Can you work these out from the model? Positions are in its coordinate system, mm. A direction names the side the tool comes from. Coordinates: 2 decimals unless noted, no trailing zeros. Order: outer loops, then holes, each group sorted by start corner. A loop starts at its lowest first (then second) coordinate and runs counter-clockwise, first axis right, second up. Notation, with made-up numbers: (-37.75, -24) - (20.25, -24) arc R21 ccw to (20.25, -7) - close; hole circle Ø4 at (74, 24). An arc over 180 degrees is marked (long way). Return JSON: item names as keys, results as strings. Group by question number.
1) Imagine slicing it at D-D (y = 0.75). Write out the boundary of the cut face in (x, z), and give its area (3 significant figures).
2) Imagine slicing it at C-C (z = 3.25). Write out the boundary of the cut face in (x, y), and give its area (3 significant figures).
3) If I drill on line 1 along X through (y, z) = (-4.25, 4.5); line 2 along Y through (x, z) = (-1.5, 6.75), over which ranges is the centre line in solid material (lowest first)?
4) For pin 1 Ø2.5 at (y, z) = (0, 3) entering from -X; pin 2 Ø0.6 at (x, y) = (6.5, 0) entering from +Z; pin 3 Ø4 at (x, z) = (2, 1.5) entering from -Y; pin 4 Ø2.5 at (y, z) = (-1.5, 3) entering from +X, each with a flat end and sliding along its axis, tell me the tip position at first contact or that it passes through.
5) Which directions (+Z, -Z, +X, -X, +Y, -Y) give clear straight access to the entire face, cutting with the end or side of a thin tool? Please do faces 1 (the face through (5.301, -3.465, 0.285)), 2 (the face through (0.1, -6.7, 0)), 3 (the face through (6.236, 1.301, 0.285)), 4 (the face through (-5.285, -3.465, 0.301)), 5 (the face through (-6.208, 1.285, 0.301)).
```python
from build123d import *
from OCP.BRepFilletAPI import BRepFilletAPI_MakeChamfer

# Parameters (mm, degrees)
SKETCH1_W           = 10
SKETCH1_H           = 10
BOSS_EXTRUDE1_DEPTH = 8
SKETCH2_W           = 14
SKETCH2_H           = 14
BOSS_EXTRUDE2_DEPTH = 2
FILLET1_R           = 2
CHAMFER1_SIZE       = 2
CHAMFER1_SIZE2      = 0.352653961
SKETCH3_W           = 2
SKETCH3_H           = 2
BOSS_EXTRUDE3_DEPTH = 1
FILLET2_R           = 1


with BuildPart() as part:
    # Sketch1 → Boss-Extrude1 (new body)
    with BuildSketch(Plane.XY):
        Rectangle(SKETCH1_W, SKETCH1_H)
    extrude(amount=BOSS_EXTRUDE1_DEPTH)

    # Sketch2 → Boss-Extrude2 (add)
    with BuildSketch(Plane(origin=(0, 0, 0), x_dir=(-1, 0, 0), z_dir=(0, 0, -1))):
        Rectangle(SKETCH2_W, SKETCH2_H)
    extrude(amount=BOSS_EXTRUDE2_DEPTH)

    # Fillet1
    fillet1_edges = [part.edges().sort_by_distance(p)[0] for p in [
        (0, 7, -2),
        (-7, 0, -2),
        (0, -7, -2),
        (7, 0, -2),
    ]]
    fillet(fillet1_edges, radius=FILLET1_R - 0.0001)  # a hair under: the kernel refuses the full size

    # Chamfer1: one chamfer whose edges measure the first distance from different faces: ONE call of the kernel's chamfer builder (chamfer() names one face for all edges)
    chamfer1_edges_1 = [part.edges().sort_by_distance(p)[0] for p in [
        (5, 0, 8),
    ]]
    chamfer1_side_1 = [part.faces().sort_by_distance(p)[0] for p in [
        (5, 0, 4),
    ]]
    chamfer1_edges_2 = [part.edges().sort_by_distance(p)[0] for p in [
        (0, 5, 8),
    ]]
    chamfer1_side_2 = [part.faces().sort_by_distance(p)[0] for p in [
        (0, 5, 4),
    ]]
    chamfer1_edges_3 = [part.edges().sort_by_distance(p)[0] for p in [
        (-5, 0, 8),
    ]]
    chamfer1_side_3 = [part.faces().sort_by_distance(p)[0] for p in [
        (-5, 0, 4),
    ]]
    chamfer1_edges_4 = [part.edges().sort_by_distance(p)[0] for p in [
        (0, -5, 8),
    ]]
    chamfer1_side_4 = [part.faces().sort_by_distance(p)[0] for p in [
        (0, -5, 4),
    ]]
    chamfer1 = BRepFilletAPI_MakeChamfer(part.part.solid().wrapped)
    for e in chamfer1_edges_1:
        chamfer1.Add(CHAMFER1_SIZE, CHAMFER1_SIZE2, e.wrapped, chamfer1_side_1[0].wrapped)  # the first distance lies on this face
    for e in chamfer1_edges_2:
        chamfer1.Add(CHAMFER1_SIZE, CHAMFER1_SIZE2, e.wrapped, chamfer1_side_2[0].wrapped)  # the first distance lies on this face
    for e in chamfer1_edges_3:
        chamfer1.Add(CHAMFER1_SIZE, CHAMFER1_SIZE2, e.wrapped, chamfer1_side_3[0].wrapped)  # the first distance lies on this face
    for e in chamfer1_edges_4:
        chamfer1.Add(CHAMFER1_SIZE, CHAMFER1_SIZE2, e.wrapped, chamfer1_side_4[0].wrapped)  # the first distance lies on this face
    add(Compound.cast(chamfer1.Shape()), mode=Mode.REPLACE)

    # Sketch3 → Boss-Extrude3 (add)
    with BuildSketch(Plane.XY):
        with Locations((-6, 0)):
            Rectangle(SKETCH3_W, SKETCH3_H)
        with Locations((6, 0)):
            Rectangle(SKETCH3_W, SKETCH3_H)
    extrude(amount=BOSS_EXTRUDE3_DEPTH)

    # Fillet2
    fillet2_edges = [part.edges().sort_by_distance(p)[0] for p in [
        (6, 1, 0),
        (6, -1, 0),
        (-6, -1, 0),
        (-6, 1, 0),
        (5, 3, 0),
        (5, -3, 0),
        (-5, 3, 0),
        (-5, -3, 0),
        (0, 5, 0),
        (0, -5, 0),
    ]]
    fillet(fillet2_edges, radius=FILLET2_R - 0.0001)  # a hair under: the kernel refuses the full size


solid = part.part
```
Calculated:
{
 "1": {"outline": "(-7, 0) arc R2 ccw to (-5, -2) - (5, -2) arc R2 ccw to (7, 0) - (7, 1) - (5, 1) - (5, 6) - (4.65, 8) - (-4.65, 8) - (-5, 6) - (-5, 1) - (-7, 1) - close", "area": "110 mm2"},
 "2": {"outline": "(-5, -5) - (5, -5) - (5, 5) - (-5, 5) - close", "area": "100 mm2"},
 "3": {"line 1": "-5 to 5", "line 2": "-4.87 to 4.87"},
 "4": {"pin 1": "x = -5", "pin 2": "z = 1", "pin 3": "y = -7", "pin 4": "x = 5"},
 "5": {"face 1": "+Z, +X, -Y", "face 2": "+Z, -Y", "face 3": "+Z, +X, +Y", "face 4": "+Z, -X, -Y", "face 5": "+Z, -X, +Y"}
}
